Design review of the part built by this model. Coordinates are the model's own, in mm. Face numbers are marked on the shaded views. A direction names the side the tool comes from. Round coordinates to 2 decimals unless told otherwise and drop trailing zeros. Loops run counter-clockwise (first coordinate to the right, second up) from the corner with the lowest first, then second, coordinate; pieces in that order, holes last. Notation, with made-up numbers: M 6,-34 L 53,-34 A22 cw 53,-5 Z; hole C 59,22 d3. An arc over 180 degrees is marked long. Use a Markdown table: item, result.
from build123d import *

# Parameters (mm, degrees)
SKETCH_1_W          = 12.25
SKETCH_1_H          = 11.3
EXTRUDE_1_DEPTH     = 2.5
SKETCH_2_W          = 1.5
SKETCH_2_H          = 11.3
EXTRUDE_2_DEPTH     = 3.85
SKETCH_5_W          = 9.25
SKETCH_5_H          = 11.5
CUT_EXTRUDE_1_DEPTH = 1
SKETCH_8_W          = 1.6
SKETCH_8_H          = 11.3
EXTRUDE_5_DEPTH     = 0.7
SKETCH_9_W          = 1.6
SKETCH_9_H          = 11.3
EXTRUDE_6_DEPTH     = 0.7
FILLET_8_R          = 0.3
SKETCH_11_W         = 12.25
SKETCH_11_H         = 4.85
CUT_EXTRUDE_2_DEPTH = 2
SKETCH_12_W         = 12.25
SKETCH_12_H         = 4.85
CUT_EXTRUDE_3_DEPTH = 2
SKETCH_13_W         = 1.5
SKETCH_13_H         = 11.3
EXTRUDE_7_DEPTH     = 0.5
SKETCH_14_W         = 1.5
SKETCH_14_H         = 11.3
EXTRUDE_8_DEPTH     = 0.5
FILLET_9_R          = 0.5
FILLET_10_R         = 0.7


with BuildPart() as part:
    # 스케치1 → 보스-돌출1 (new body)
    with BuildSketch(Plane.XY):
        Rectangle(SKETCH_1_W, SKETCH_1_H)
    extrude(amount=EXTRUDE_1_DEPTH)

    # 스케치2 → 보스-돌출2 (add)
    with BuildSketch(Plane.XY.offset(2.5)):
        with Locations((-5.375, 0)):
            Rectangle(SKETCH_2_W, SKETCH_2_H)
        with Locations((5.375, 0)):
            Rectangle(SKETCH_2_W, SKETCH_2_H)
    extrude(amount=EXTRUDE_2_DEPTH)

    # 스케치5 → 컷-돌출1 (cut)
    with BuildSketch(Plane.XY.offset(2.5)):
        Rectangle(SKETCH_5_W, SKETCH_5_H)
    extrude(amount=-CUT_EXTRUDE_1_DEPTH, mode=Mode.SUBTRACT)

    # 스케치8 → 보스-돌출5 (add)
    with BuildSketch(Plane(origin=(-4.625, 0, 0), x_dir=(0, 0, -1), z_dir=(1, 0, 0))):
        with Locations((-5.55, 0)):
            Rectangle(SKETCH_8_W, SKETCH_8_H)
    extrude(amount=EXTRUDE_5_DEPTH)

    # 스케치9 → 보스-돌출6 (add)
    with BuildSketch(Plane.ZY.offset(-4.625)):
        with Locations((5.55, 0)):
            Rectangle(SKETCH_9_W, SKETCH_9_H)
    extrude(amount=EXTRUDE_6_DEPTH)

    # 필렛8
    fillet_8_edges = [part.edges().sort_by_distance(p)[0] for p in [
        (4.625, 0, 1.5),
        (-4.625, 0, 1.5),
    ]]
    fillet(fillet_8_edges, radius=FILLET_8_R)

    # 스케치11 → 컷-돌출2 (cut)
    with BuildSketch(Plane(origin=(0, 5.65, 0), x_dir=(1, 0, 0), z_dir=(0, 1, 0))):
        with Locations((0, -3.925)):
            Rectangle(SKETCH_11_W, SKETCH_11_H)
    extrude(amount=-CUT_EXTRUDE_2_DEPTH, mode=Mode.SUBTRACT)

    # 스케치12 → 컷-돌출3 (cut)
    with BuildSketch(Plane.XZ.offset(5.65)):
        with Locations((0, 3.925)):
            Rectangle(SKETCH_12_W, SKETCH_12_H)
    extrude(amount=-CUT_EXTRUDE_3_DEPTH, mode=Mode.SUBTRACT)

    # 스케치13 → 보스-돌출7 (add)
    with BuildSketch(Plane(origin=(6.125, 0, 0), x_dir=(0, 0, -1), z_dir=(1, 0, 0))):
        with Locations((-0.75, 0)):
            Rectangle(SKETCH_13_W, SKETCH_13_H)
    extrude(amount=EXTRUDE_7_DEPTH)

    # 스케치14 → 보스-돌출8 (add)
    with BuildSketch(Plane.ZY.offset(6.125)):
        with Locations((0.75, 0)):
            Rectangle(SKETCH_14_W, SKETCH_14_H)
    extrude(amount=EXTRUDE_8_DEPTH)

    # 필렛9
    fillet_9_edges = [part.edges().sort_by_distance(p)[0] for p in [
        (6.125, 0, 1.5),
        (-6.125, 0, 1.5),
    ]]
    fillet(fillet_9_edges, radius=FILLET_9_R - 0.0001)  # a hair under: the kernel refuses the full size

    # 필렛10
    fillet_10_edges = [part.edges().sort_by_distance(p)[0] for p in [
        (-3.925, 0, 6.35),
        (-3.925, 0, 4.75),
        (3.925, 0, 4.75),
        (3.925, 0, 6.35),
    ]]
    fillet(fillet_10_edges, radius=FILLET_10_R - 0.0001)  # a hair under: the kernel refuses the full size


solid = part.part
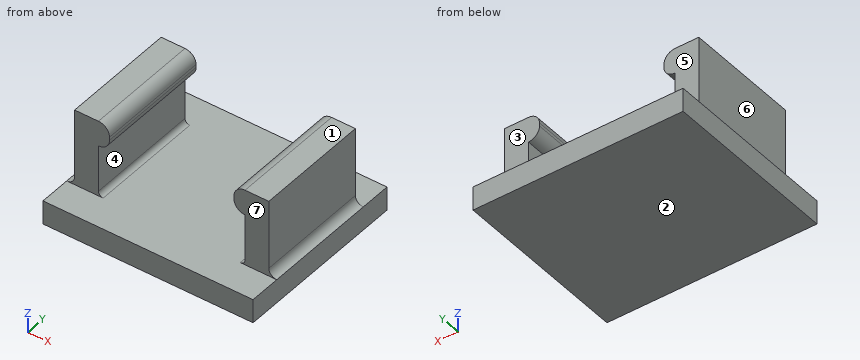
1. Take a section at B-B on x = 5.75. Give the boundary of the cut face in (y, z).
Check values:
| item | result |
|---|---|
| outline | M -5.65,0 L 5.65,0 L 5.65,1.5 L 3.65,1.5 L 3.65,6.35 L -3.65,6.35 L -3.65,1.5 L -5.65,1.5 Z |
2. Wall thickness on line 1 along X through (y, z) = (-0.25, 3.5) (3 decimals); line 2 along Z through (x, y) = (1.5, -5); line 3 along X through (y, z) = (3, 6) (3 decimals): over which ranges is each line inside the solid? List them lowest first. Write a range as from..to.
Check values:
| item | result |
|---|---|
| line 1 | x = -6.125..-4.625, 4.625..6.125 |
| line 2 | z = 0..1.5 |
| line 3 | x = -6.125..-4.019, 4.019..6.125 |
3. Take a section at A-A on z = 4.25. Give the boundary of the cut face in (x, y) (3 decimals).
Check values:
| item | result |
|---|---|
| outline | M -6.125,-3.65 L -4.625,-3.65 L -4.625,3.65 L -6.125,3.65 Z; M 4.625,-3.65 L 6.125,-3.65 L 6.125,3.65 L 4.625,3.65 Z |
4. Insertion check: pin 1 (3 mm diameter, centred on x = -5, y = 0.5, fed in from -Z); pin 2 (2.5 mm diameter, centred on y = 0, z = 3.5, fed in from -X) (3 decimals); pin 3 (0.8 mm diameter, centred on x = 5, z = 5, fed in from -Y); pin 4 (1.3 mm diameter, centred on y = 0.5, z = 5, fed in from +X) (3 decimals). Each pin has a flat end and moves straight along its axis. Give the tip position at first contact, or say it passes through.
Check values:
| item | result |
|---|---|
| pin 1 | stops at z = 0 |
| pin 2 | stops at x = -6.125 |
| pin 3 | stops at y = -3.65 |
| pin 4 | stops at x = 6.125 |
5. The part is to be moulded in two halves that separate along Z. For the marked faces 1, 2, 3 and 4, say which applies: pulls with the +Z half, pulls with the -Z half, needs draft (parallel to the pull), parting line crosses it, or undercut.
Check values:
| item | result |
|---|---|
| face 1 | pulls with the +Z half |
| face 2 | pulls with the -Z half |
| face 3 | needs draft |
| face 4 | undercut |
6. Machinability: for the marked faces 5, 6 and 7, which of the approach directions +Z, -Z, +X, -X, +Y, -Y give a long, thin tool a straight path to every point of the face, cutting with its end or side? Answer none if there is none.
Check values:
| item | result |
|---|---|
| face 5 | +Z, +X, -X, +Y |
| face 6 | +Z, -X, +Y, -Y |
| face 7 | +Z, +X, -X, -Y |
7. Take a section at D-D on z = 5.25. Give the boundary of the cut face in (x, y) (3 decimals).
Check values:
| item | result |
|---|---|
| outline | M -6.125,-3.65 L -3.954,-3.65 L -3.954,3.65 L -6.125,3.65 Z; M 3.954,-3.65 L 6.125,-3.65 L 6.125,3.65 L 3.954,3.65 Z |
